from build123d import *

# Parameters (mm, degrees)
BOSS_EXTRUDE1_DEPTH            = 6.35
F_5_16_0_3125_DIAMETER_HOLE1_D = 7.9375
F_5_16_0_3125_DIAMETER_HOLE2_D = 7.9375


with BuildPart() as part:
    # Sketch1 → Boss-Extrude1 (new body, symmetric)
    with BuildSketch(Plane.XY):
        Polygon((0, 0), (0, 25.4), (-1, 25.4), (-1, 1), (-25.4, 1), (-25.4, 0), align=None)
    extrude(amount=BOSS_EXTRUDE1_DEPTH, both=True)

    # 5/16 (0.3125) Diameter Hole1 (through all)
    with Locations(Plane.ZY.offset(1)):
        with Locations((0, 13.2)):
            Hole(F_5_16_0_3125_DIAMETER_HOLE1_D / 2)

    # 5/16 (0.3125) Diameter Hole2 (through all)
    with Locations(Plane(origin=(-13.2, 1, 0), x_dir=(1, 0, 0), z_dir=(0, 1, 0))):
        with Locations((0, 0)):
            Hole(F_5_16_0_3125_DIAMETER_HOLE2_D / 2)


solid = part.part
Design review of the part built by this model. Coordinates are the model's own, in mm. A direction names the side the tool comes from. Give positions to 0.01 mm unless a question says otherwise; leave off trailing zeros. Write each loop counter-clockwise with the first axis right and the second up, starting at its lowest first coordinate (ties: lowest second). Pieces come first, ordered by that corner, then holes. Notation, with made-up numbers: M 11,82 L 26,82 A22 ccw 26,90 Z; hole C 38,55 d9. An arc over 180 degrees is marked long. Answer as a JSON object with one key per item and string values. Group by question number.
1) Tool access review of faces 4 (the face through (-0.5, 25.4, 0.1)), 5 (the face through (-1, 13.4, 4.3)): name each direction out of +Z, -Z, +X, -X, +Y, -Y from which nothing blocks a thin tool from reaching the whole face with its end or side.
2) Clearance check with flat-ended pins moving along their axes: pin 1 Ø6.5 at (x, z) = (-13.2, 0) entering from +Y; pin 2 Ø5 at (y, z) = (10.5, -2) entering from -X; pin 3 Ø4 at (x, z) = (-11, 1.5) entering from +Y. State where each tip first meets the part, or that it passes through.
3) For line 1 along Z through (x, y) = (-13.2, 0.4); line 2 along Y through (x, z) = (-0.15, 0); line 3 along X through (y, z) = (4, 5.75), list the stretches that pass through material, from the lowest coordinate up.
4) Mouldability with a two-part tool opening along Y and no side actions: class faces 1 (the face through (-7.1, 0.5, 6.35)), 2 (the face through (-10, 1, -3)), 3 (the face through (-0.493, 9.326, 0.86)) as released by +Y, released by -Y, zero draft, split by the parting line, or undercut.
5) We need section D-D (z = -2.5). Give the boundary of the cut face in (x, y).
6) We need section A-A (z = 0). Give the boundary of the cut face in (x, y).
7) We need section B-B (y = 13.2). Give the boundary of the cut face in (x, z), and give its area (3 significant figures).
8) We need section C-C (x = -13.2). Give the boundary of the cut face in (y, z).
Answer key:
{
 "1": {"face 4": "+Z, -Z, +X, -X, +Y", "face 5": "+Z, -Z, -X, +Y"},
 "2": {"pin 1": "passes through", "pin 2": "stops at x = -1", "pin 3": "stops at y = 1"},
 "3": {"line 1": "z = -6.35 to -3.97, 3.97 to 6.35", "line 2": "y = 0 to 9.23, 17.17 to 25.4", "line 3": "x = -1 to 0"},
 "4": {"face 1": "zero draft", "face 2": "released by +Y", "face 3": "undercut"},
 "5": {"outline": "M -25.4,0 L -16.28,0 L -16.28,1 L -25.4,1 Z; M -10.12,0 L 0,0 L 0,10.12 L -1,10.12 L -1,1 L -10.12,1 Z; M -1,16.28 L 0,16.28 L 0,25.4 L -1,25.4 Z"},
 "6": {"outline": "M -25.4,0 L -17.17,0 L -17.17,1 L -25.4,1 Z; M -9.23,0 L 0,0 L 0,9.23 L -1,9.23 L -1,1 L -9.23,1 Z; M -1,17.17 L 0,17.17 L 0,25.4 L -1,25.4 Z"},
 "7": {"outline": "M -1,-6.35 L 0,-6.35 L 0,-3.97 L -1,-3.97 Z; M -1,3.97 L 0,3.97 L 0,6.35 L -1,6.35 Z", "area": "4.76 mm²"},
 "8": {"outline": "M 0,-6.35 L 1,-6.35 L 1,-3.97 L 0,-3.97 Z; M 0,3.97 L 1,3.97 L 1,6.35 L 0,6.35 Z"}
}
